Read the model definition and answer for the solid it produces. Units are mm, in the model's axes. A direction names the side the tool comes from. Coordinates: 2 decimals unless noted, no trailing zeros. Write each loop counter-clockwise with the first axis right and the second up, starting at its lowest first coordinate (ties: lowest second). Pieces come first, ordered by that corner, then holes.
Item 1: Determine the mould class of faces 1 (the face through (79.048, -2.306, 5.287)), 2 (the face through (1, -1, -17.5)), 3 (the face through (-5.25, 2.46, -39.64)) for opening direction X: released by +X, released by -X, zero draft, split by the parting line, or undercut.
Item 2: Section A-A (z = -55.1) is taken. Give the vertices of the cut face in (x, y) (3 decimals), then the cut area to 3 significant figures.
Item 3: A tool of negligible diameter and unlimited length cuts with its end or side. For faces 4 (the face through (4, 1, -12)), 5 (the face through (39.15, -4, 2)), 6 (the face through (5, -1, 1)), from which of +Z, -Z, +X, -X, +Y, -Y can it reach the whole face along a straight path? Write none if from no direction.
Item 4: Straight lines are drawn through the part: probe 1 along X at (y, z) = (-1.1, -12.5); probe 2 along X at (y, z) = (0.25, -2.5); probe 3 along X at (y, z) = (-1.25, -60.5). For each, find the intervals that lie inside material, in ascending order.
Item 5: Each of these flat-tipped pins is pushed along its axis until it touches: P1, Ø5, axis at x = 31, y = -6.5, coming from the +Z side; P2, Ø1.5, axis at x = 71, z = -65.5, coming from the -Y side; P3, Ø1.4, axis at y = -4.5, z = 5, coming from the -X side. Where does it stop, or does it pass through?
Item 6: Section B-B (x = 43.5) is taken. Give the vertices of the cut face in (y, z) (3 decimals).
from build123d import *

# Parameters (mm, degrees)
SKETCH1_W           = 85.8
SKETCH1_H           = 92.5
SKETCH1_R           = 2.05
BOSS_EXTRUDE1_DEPTH = 3.175
SKETCH2_W           = 85.8
SKETCH2_H           = 92.5
SKETCH2_R           = 1.35
SKETCH2_R_2         = 3.35
BOSS_EXTRUDE2_DEPTH = 1.905
BOSS_EXTRUDE3_START = 1
SKETCH2_3_W         = 85.8
SKETCH2_3_H         = 92.5
SKETCH2_3_R         = 1.35
SKETCH2_3_R_2       = 3.35
BOSS_EXTRUDE3_DEPTH = 1
SKETCH3_W           = 85.8
SKETCH3_H           = 92.5
SKETCH3_W_2         = 75.8
SKETCH3_H_2         = 82.5
BOSS_EXTRUDE4_DEPTH = 3.3
SKETCH4_W           = 14
SKETCH4_H           = 6.75
CUT_EXTRUDE1_DEPTH  = 118.802300593
SKETCH5_W           = 10
SKETCH5_H           = 6
CUT_EXTRUDE2_DEPTH  = 118.802300593
BOSS_EXTRUDE5_DEPTH = 3.5
FILLET1_R           = 2.5
FILLET2_R           = 2.5
FILLET3_R           = 2.5
FILLET4_R           = 2.5
FILLET5_R           = 2.5
CUT_EXTRUDE3_DEPTH  = 3.36
CUT_EXTRUDE4_DEPTH  = 75
SKETCH10_W          = 4.501
SKETCH10_H          = 2
BOSS_EXTRUDE6_DEPTH = 5
SKETCH13_R          = 6.35
CUT_EXTRUDE5_DEPTH  = 2.5


with BuildPart() as part:
    # Sketch1 → Boss-Extrude1 (new body)
    with BuildSketch(Plane(origin=(0, 0, 0), x_dir=(1, 0, 0), z_dir=(0, 1, 0))):
        with Locations((36.9, 40.25)):
            Rectangle(SKETCH1_W, SKETCH1_H)
        with Locations(Location((2.5, 12.5, 0), (0, 0, 270))):
            Circle(SKETCH1_R, mode=Mode.SUBTRACT)
        with Locations(Location((18.4, 2.5, 0), (0, 0, 270))):
            Circle(SKETCH1_R, mode=Mode.SUBTRACT)
        with Locations(Location((36.9, 2.5, 0), (0, 0, 270))):
            Circle(SKETCH1_R, mode=Mode.SUBTRACT)
        with Locations(Location((55.4, 2.5, 0), (0, 0, 270))):
            Circle(SKETCH1_R, mode=Mode.SUBTRACT)
        with Locations(Location((29.3, 55.1, 0), (0, 0, 270))):
            Circle(SKETCH1_R, mode=Mode.SUBTRACT)
        with Locations(Location((70.8, 74.5, 0), (0, 0, 270))):
            Circle(SKETCH1_R, mode=Mode.SUBTRACT)
    extrude(amount=BOSS_EXTRUDE1_DEPTH)

    # Sketch2 → Boss-Extrude2 (add)
    # profile 1 of 2: a face of its own
    with BuildSketch(Plane(origin=(0, 0, 0), x_dir=(1, 0, 0), z_dir=(0, 1, 0))):
        with Locations((36.9, 40.25)):
            Rectangle(SKETCH2_W, SKETCH2_H)
        with Locations(Location((2.5, 12.5, 0), (0, 0, 270))):
            Circle(SKETCH2_R, mode=Mode.SUBTRACT)
        with Locations(Location((18.4, 2.5, 0), (0, 0, 270))):
            Circle(SKETCH2_R, mode=Mode.SUBTRACT)
        with Locations(Location((36.9, 2.5, 0), (0, 0, 270))):
            Circle(SKETCH2_R, mode=Mode.SUBTRACT)
        with Locations(Location((55.4, 2.5, 0), (0, 0, 270))):
            Circle(SKETCH2_R, mode=Mode.SUBTRACT)
        with Locations(Location((70.8, 74.5, 0), (0, 0, 270))):
            Circle(SKETCH2_R, mode=Mode.SUBTRACT)
        with BuildLine():
            Line((65.8, 74.5), (65.8, 81.5))
            Line((65.8, 81.5), (-1, 81.5))
            Line((-1, 81.5), (-1, 17.5))
            Line((-1, 17.5), (2.5, 17.5))
            ThreePointArc((2.5, 17.5), (7.5, 12.5), (2.5, 7.5))
            Line((2.5, 7.5), (-1, 7.5))
            Line((-1, 7.5), (-1, -1))
            Line((-1, -1), (13.4, -1))
            Line((13.4, -1), (13.4, 2.5))
            ThreePointArc((13.4, 2.5), (18.4, 7.5), (23.4, 2.5))
            Line((23.4, 2.5), (23.4, -1))
            Line((23.4, -1), (31.9, -1))
            Line((31.9, -1), (31.9, 2.5))
            ThreePointArc((31.9, 2.5), (36.9, 7.5), (41.9, 2.5))
            Line((41.9, 2.5), (41.9, -1))
            Line((41.9, -1), (50.4, -1))
            Line((50.4, -1), (50.4, 2.5))
            ThreePointArc((50.4, 2.5), (55.4, 7.5), (60.4, 2.5))
            Line((60.4, 2.5), (60.4, -1))
            Line((60.4, -1), (74.8, -1))
            Line((74.8, -1), (74.8, 69.5))
            Line((74.8, 69.5), (70.8, 69.5))
            ThreePointArc((70.8, 69.5), (67.264466094, 70.964466094), (65.8, 74.5))
        make_face(mode=Mode.SUBTRACT)
    # profile 2 of 2: a face of its own
    with BuildSketch(Plane(origin=(0, 0, 0), x_dir=(1, 0, 0), z_dir=(0, 1, 0))):
        with Locations(Location((29.3, 55.1, 0), (0, 0, 270))):
            Circle(SKETCH2_R_2)
        with Locations(Location((29.3, 55.1, 0), (0, 0, 270))):
            Circle(SKETCH2_R, mode=Mode.SUBTRACT)
    extrude(amount=-BOSS_EXTRUDE2_DEPTH)

    # Sketch2_3 → Boss-Extrude3 (add)
    # profile 1 of 2: a face of its own
    with BuildSketch(Plane(origin=(0, 0, 0), x_dir=(1, 0, 0), z_dir=(0, 1, 0)).offset(BOSS_EXTRUDE3_START)):
        with Locations((36.9, 40.25)):
            Rectangle(SKETCH2_3_W, SKETCH2_3_H)
        with Locations(Location((2.5, 12.5, 0), (0, 0, 270))):
            Circle(SKETCH2_3_R, mode=Mode.SUBTRACT)
        with Locations(Location((18.4, 2.5, 0), (0, 0, 270))):
            Circle(SKETCH2_3_R, mode=Mode.SUBTRACT)
        with Locations(Location((36.9, 2.5, 0), (0, 0, 270))):
            Circle(SKETCH2_3_R, mode=Mode.SUBTRACT)
        with Locations(Location((55.4, 2.5, 0), (0, 0, 270))):
            Circle(SKETCH2_3_R, mode=Mode.SUBTRACT)
        with Locations(Location((70.8, 74.5, 0), (0, 0, 270))):
            Circle(SKETCH2_3_R, mode=Mode.SUBTRACT)
        with BuildLine():
            Line((65.8, 74.5), (65.8, 81.5))
            Line((65.8, 81.5), (-1, 81.5))
            Line((-1, 81.5), (-1, 17.5))
            Line((-1, 17.5), (2.5, 17.5))
            ThreePointArc((2.5, 17.5), (7.5, 12.5), (2.5, 7.5))
            Line((2.5, 7.5), (-1, 7.5))
            Line((-1, 7.5), (-1, -1))
            Line((-1, -1), (13.4, -1))
            Line((13.4, -1), (13.4, 2.5))
            ThreePointArc((13.4, 2.5), (18.4, 7.5), (23.4, 2.5))
            Line((23.4, 2.5), (23.4, -1))
            Line((23.4, -1), (31.9, -1))
            Line((31.9, -1), (31.9, 2.5))
            ThreePointArc((31.9, 2.5), (36.9, 7.5), (41.9, 2.5))
            Line((41.9, 2.5), (41.9, -1))
            Line((41.9, -1), (50.4, -1))
            Line((50.4, -1), (50.4, 2.5))
            ThreePointArc((50.4, 2.5), (55.4, 7.5), (60.4, 2.5))
            Line((60.4, 2.5), (60.4, -1))
            Line((60.4, -1), (74.8, -1))
            Line((74.8, -1), (74.8, 69.5))
            Line((74.8, 69.5), (70.8, 69.5))
            ThreePointArc((70.8, 69.5), (67.264466094, 70.964466094), (65.8, 74.5))
        make_face(mode=Mode.SUBTRACT)
    # profile 2 of 2: a face of its own
    with BuildSketch(Plane(origin=(0, 0, 0), x_dir=(1, 0, 0), z_dir=(0, 1, 0)).offset(BOSS_EXTRUDE3_START)):
        with Locations(Location((29.3, 55.1, 0), (0, 0, 270))):
            Circle(SKETCH2_3_R_2)
        with Locations(Location((29.3, 55.1, 0), (0, 0, 270))):
            Circle(SKETCH2_3_R, mode=Mode.SUBTRACT)
    extrude(amount=-BOSS_EXTRUDE3_DEPTH)

    # Sketch3 → Boss-Extrude4 (add)
    with BuildSketch(Plane(origin=(0, -1.905, 0), x_dir=(-1, 0, 0), z_dir=(0, -1, 0))):
        with Locations((-36.9, 40.25)):
            Rectangle(SKETCH3_W, SKETCH3_H)
        with Locations((-36.9, 40.25)):
            Rectangle(SKETCH3_W_2, SKETCH3_H_2, mode=Mode.SUBTRACT)
    extrude(amount=BOSS_EXTRUDE4_DEPTH)

    # Sketch4 → Cut-Extrude1 (cut, through all)
    with BuildSketch(Plane.XY):
        with Locations((9.15, -5.22)):
            Rectangle(SKETCH4_W, SKETCH4_H)
        with Locations((27.65, -5.22)):
            Rectangle(SKETCH4_W, SKETCH4_H)
        with Locations((46.15, -5.22)):
            Rectangle(SKETCH4_W, SKETCH4_H)
        with Locations((64.65, -5.22)):
            Rectangle(SKETCH4_W, SKETCH4_H)
    extrude(amount=CUT_EXTRUDE1_DEPTH, mode=Mode.SUBTRACT)

    # Sketch5 → Cut-Extrude2 (cut, through all)
    with BuildSketch(Plane.XY):
        with Locations((58, -6.205)):
            Rectangle(SKETCH5_W, SKETCH5_H)
    extrude(amount=-CUT_EXTRUDE2_DEPTH, mode=Mode.SUBTRACT)

    # Sketch6 → Boss-Extrude5 (add)
    with BuildSketch(Plane.ZY.offset(6)):
        with BuildLine():
            Line((-59.6, 0), (-59.6, -8.5))
            Line((-59.6, -8.5), (-59.131128874, -8.5))
            ThreePointArc((-59.131128874, -8.5), (-55.1, -6), (-51.068871126, -8.5))
            Line((-51.068871126, -8.5), (-50.6, -8.5))
            Line((-50.6, -8.5), (-50.6, 0))
            Line((-50.6, 0), (-59.6, 0))
        make_face()
    extrude(amount=-BOSS_EXTRUDE5_DEPTH)

    # Fillet1
    fillet1_edges = [part.edges().sort_by_distance(p)[0] for p in [
        (79.8, -1.015, 6),
    ]]
    fillet(fillet1_edges, radius=FILLET1_R)

    # Fillet2
    fillet2_edges = [part.edges().sort_by_distance(p)[0] for p in [
        (79.8, -1.015, -86.5),
    ]]
    fillet(fillet2_edges, radius=FILLET2_R)

    # Fillet3
    fillet3_edges = [part.edges().sort_by_distance(p)[0] for p in [
        (-6, -1.015, -86.5),
    ]]
    fillet(fillet3_edges, radius=FILLET3_R)

    # Fillet4
    fillet4_edges = [part.edges().sort_by_distance(p)[0] for p in [
        (-6, -1.015, 6),
    ]]
    fillet(fillet4_edges, radius=FILLET4_R)

    # Fillet5
    fillet5_edges = [part.edges().sort_by_distance(p)[0] for p in [
        (79.8, 3.175, -40.25),
        (79.067766953, 3.175, 5.267766953),
        (36.9, 3.175, -86.5),
        (79.067766953, 3.175, -85.767766953),
        (-6, 3.175, -40.25),
        (-5.267766953, 3.175, -85.767766953),
        (36.9, 3.175, 6),
        (-5.267766953, 3.175, 5.267766953),
    ]]
    fillet(fillet5_edges, radius=FILLET5_R)

    # Sketch7 → Cut-Extrude3 (cut)
    with BuildSketch(Plane(origin=(0, -5.205, 0), x_dir=(-1, 0, 0), z_dir=(0, -1, 0))):
        Polygon((-2.15, -2.75), (-0.4, -3.75), (-2.15, -4.75), align=None)
        Polygon((-16.15, -2.75), (-17.9, -3.75), (-16.15, -4.75), align=None)
        Polygon((-20.65, -2.75), (-18.9, -3.75), (-20.65, -4.75), align=None)
        Polygon((-34.65, -2.75), (-36.4, -3.75), (-34.65, -4.75), align=None)
        Polygon((-39.15, -2.75), (-39.15, -4.75), (-37.4, -3.75), align=None)
        Polygon((-53.15, -2.75), (-53.15, -4.75), (-54.9, -3.75), align=None)
        Polygon((-57.65, -4.75), (-55.9, -3.75), (-57.65, -2.75), align=None)
        Polygon((-71.65, -2.75), (-73.4, -3.75), (-71.65, -4.75), align=None)
    extrude(amount=-CUT_EXTRUDE3_DEPTH, mode=Mode.SUBTRACT)

    # Sketch8 → Cut-Extrude4 (cut)
    with BuildSketch(Plane(origin=(0, 0, 0), x_dir=(0, 0, -1), z_dir=(1, 0, 0))):
        Polygon((-4.75, -1.9), (-2.75, -1.9), (-3.75, -0.15), align=None)
    extrude(amount=CUT_EXTRUDE4_DEPTH, mode=Mode.SUBTRACT)

    # Sketch10 → Boss-Extrude6 (add)
    with BuildSketch(Plane.XY.offset(6)):
        with Locations((-0.1005, -0.845)):
            Rectangle(SKETCH10_W, SKETCH10_H)
        with Locations((18.3995, -0.845)):
            Rectangle(SKETCH10_W, SKETCH10_H)
        with Locations((36.8995, -0.845)):
            Rectangle(SKETCH10_W, SKETCH10_H)
        with Locations((55.3995, -0.845)):
            Rectangle(SKETCH10_W, SKETCH10_H)
        with Locations((73.9005, -0.845)):
            Rectangle(SKETCH10_W, SKETCH10_H)
    extrude(amount=-BOSS_EXTRUDE6_DEPTH)

    # Sketch13 → Cut-Extrude5 (cut)
    with BuildSketch(Plane(origin=(0, 0, 0), x_dir=(0, 0, -1), z_dir=(1, 0, 0))):
        with Locations((55.1, -10.95)):
            Circle(SKETCH13_R)
    extrude(amount=-CUT_EXTRUDE5_DEPTH, mode=Mode.SUBTRACT)


solid = part.part
Established:
1. face 1: released by +X
1. face 2: undercut
1. face 3: released by -X
2. outline: (-6, -6) - (-2.5, -6) - (-2.5, -4.6) - (-1, -4.6) - (-1, 0) - (25.95, 0) - (25.95, -1.905) - (27.95, -1.905) - (27.95, 1) - (27.25, 1) - (27.25, 3.175) - (-3.5, 3.175) arc R2.5 ccw to (-6, 0.675) - close; (30.65, -1.905) - (32.65, -1.905) - (32.65, 0) - (74.8, 0) - (74.8, -5.205) - (79.8, -5.205) - (79.8, 0.675) arc R2.5 ccw to (77.3, 3.175) - (31.35, 3.175) - (31.35, 1) - (30.65, 1) - close
2. area: 320 mm2
3. face 4: +Y
3. face 5: +Z, -Y
3. face 6: -Y
4. probe 1: x = -6 to 1.15, 3.85 to 7.5, 74.8 to 79.8
4. probe 2: x = -6 to 17.05, 19.75 to 35.55, 38.25 to 54.05, 56.75 to 79.8
4. probe 3: x = -6 to -1, 74.8 to 79.8
5. P1: stops at z = -81.5
5. P2: stops at y = 0
5. P3: stops at x = -5.87
6. outline: (-5.205, -86.5) - (0.675, -86.5) arc R2.5 ccw to (3.175, -84) - (3.175, 3.5) arc R2.5 ccw to (0.675, 6) - (-1.845, 6) - (-1.845, 4.719) - (-0.15, 3.75) - (-1.845, 2.781) - (-1.845, 1) - (0, 1) - (0, -81.5) - (-5.205, -81.5) - close
